Model file for the job. Use its own axes, mm. A direction names the side the tool comes from. Round coordinates to 2 decimals unless told otherwise and drop trailing zeros. Write each loop counter-clockwise with the first axis right and the second up, starting at its lowest first coordinate (ties: lowest second). Pieces come first, ordered by that corner, then holes.
```python
from build123d import *

# Parameters (mm, degrees)
SKETCH2_R           = 2.5
BOSS_EXTRUDE1_DEPTH = 5
FILLET1_R           = 1.1
SKETCH5_R           = 2.5
BOSS_EXTRUDE2_DEPTH = 5


with BuildPart() as part:
    # Sketch2 → Boss-Extrude1 (new body)
    with BuildSketch(Plane.XY):
        with BuildLine():
            Line((-8.409252233, 1.684959921), (-4.836047922, -18.148987446))
            ThreePointArc((-4.836047922, -18.148987446), (0, -22.191645553), (4.836047922, -18.148987446))
            Line((4.836047922, -18.148987446), (8.409252233, 1.684959921))
            ThreePointArc((8.409252233, 1.684959921), (0, 11.744565684), (-8.409252233, 1.684959921))
        make_face()
        with Locations((0, 3.199937034)):
            Circle(SKETCH2_R, mode=Mode.SUBTRACT)
    extrude(amount=BOSS_EXTRUDE1_DEPTH)

    # Fillet1
    fillet1_edges = [part.edges().sort_by_distance(p)[0] for p in [
        (0, -22.191645553, 5),
        (-2.5, 3.199937034, 0),
        (-2.5, 3.199937034, 5),
        (6.622650078, -8.232013763, 5),
        (0, 11.744565684, 5),
        (6.622650078, -8.232013763, 0),
        (0, -22.191645553, 0),
        (-6.622650078, -8.232013763, 0),
        (0, 11.744565684, 0),
        (-6.622650078, -8.232013763, 5),
    ]]
    fillet(fillet1_edges, radius=FILLET1_R)

    # Sketch5 → Boss-Extrude2 (add)
    with BuildSketch(Plane.XY.offset(5)):
        with Locations(Location((0, -17.825950176, 0), (0, 0, 180))):
            Circle(SKETCH5_R)
    extrude(amount=BOSS_EXTRUDE2_DEPTH)


solid = part.part
```
1) Cut at A-A on x = 0. List the corners of the cut face in (y, z), and give its area (3 significant figures).
2) Which spindle directions (+Z, -Z, +X, -X, +Y, -Y) get a long thin tool onto all of the face, cutting with end or side? Do faces 4 (the face through (0.325, -20.305, 7.465)), 5 (the face through (6.34, -8.04, 0.33)). Say none if no direction does.
3) Cut at B-B on z = 3.5. List the corners of the cut face in (x, y), and give its area (3 significant figures).
4) Flat gauge pins, fed straight in: pin 1 Ø5 at (y, z) = (-5, 2) entering from -X; pin 2 Ø7.5 at (x, y) = (1, -9.5) entering from +Z; pin 3 Ø6 at (x, z) = (-5, 1.5) entering from -Y. Where does each tip first touch, or does it go through?
5) Wall check: probe 1 along Y at (x, z) = (0, 3.35); probe 2 along Z at (x, y) = (6, 2); probe 3 along Y at (x, z) = (-1.5, 2.75). Give the ranges that are in metal, low to high.
6) Cut at C-C on z = 5.5. List the corners of the cut face in (x, y), and give its area (3 significant figures).
7) Pull direction X, two halves, no side cores. Call faces 1 (the face through (-0.1, -22.19, 2.48)), 2 (the face through (1.34, 5.31, 2.48)), 3 (the face through (6.598, -8.371, 2.48)): released by +X, released by -X, zero draft, split by the parting line, or undercut.
Result sheet:
1. outline: (-22.19, 1.1) arc R1.1 ccw to (-21.09, 0) - (-0.4, 0) arc R1.1 ccw to (0.7, 1.1) - (0.7, 3.9) arc R1.1 ccw to (-0.4, 5) - (-15.33, 5) - (-15.33, 10) - (-20.33, 10) - (-20.33, 5) - (-21.09, 5) arc R1.1 ccw to (-22.19, 3.9) - close; (5.7, 1.1) arc R1.1 ccw to (6.8, 0) - (10.64, 0) arc R1.1 ccw to (11.74, 1.1) - (11.74, 3.9) arc R1.1 ccw to (10.64, 5) - (6.8, 5) arc R1.1 ccw to (5.7, 3.9) - close
1. area: 168 mm2
2. face 4: +Z
2. face 5: -Z, +X, -Y
3. outline: (-8.41, 1.68) - (-4.84, -18.15) arc R4.91 ccw to (4.84, -18.15) - (8.41, 1.68) arc R8.54 ccw (long way) to start; hole circle Ø5 at (0, 3.2)
3. area: 413 mm2
4. pin 1: stops at x = -7.66
4. pin 2: stops at z = 5
4. pin 3: stops at y = -21.77
5. probe 1: y = -22.19 to 0.7, 5.7 to 11.74
5. probe 2: z = 0 to 5
5. probe 3: y = -21.96 to 1.2, 5.2 to 11.61
6. outline: circle Ø5 at (0, -17.83)
6. area: 19.6 mm2
7. face 1: split by the parting line
7. face 2: undercut
7. face 3: released by +X
